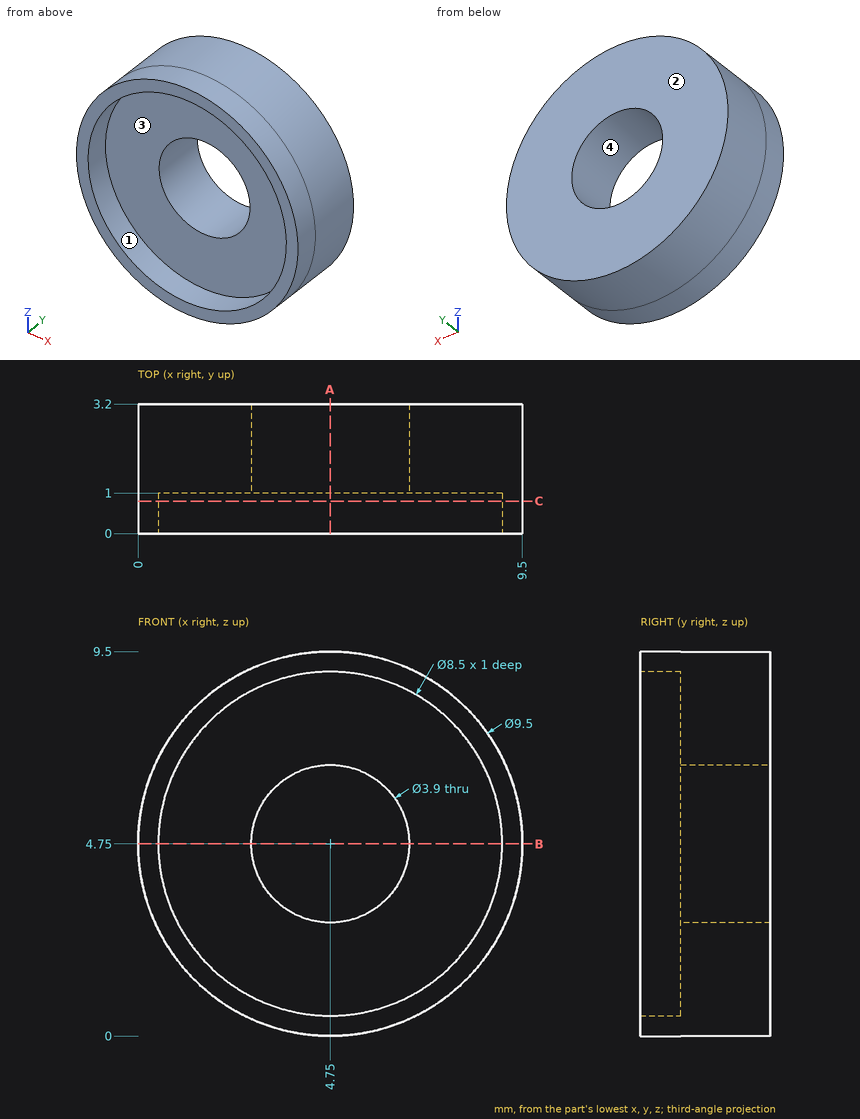
Check sheet for the drawn part. Datum: minimum x, y, z corner. Units: mm. A direction names the side the tool comes from. Round coordinates to 2 decimals unless told otherwise and drop trailing zeros. Loops run counter-clockwise (first coordinate to the right, second up) from the corner with the lowest first, then second, coordinate; pieces in that order, holes last. Notation, with made-up numbers: M 35.25,17.25 L 84.25,17.25 A27 ccw 84.25,36.25 Z; hole C 11,8.25 d7. An arc over 180 degrees is marked long. One line per question, with ' | ' between items. Start each with the question number.
Item 1: Scan lines: probe 1 along X at (y, z) = (0.4, 4.75); probe 2 along X at (y, z) = (1.5, 4.75); probe 3 along Y at (x, z) = (2.5, 7.75). Record each from-to range of solid material in increasing order.
Item 2: Release check for a two-part mould opening along X. For the marked faces 1 and 2 record: released by +X, released by -X, zero draft, split by the parting line, or undercut.
Item 3: Gauge pin test, flat ends, axial feed: pin 1 Ø1 at (x, y) = (7.5, 0.5) entering from +Z; pin 2 Ø3.5 at (x, z) = (4.75, 4.75) entering from -Y. Record the tip position at first contact, or that the pin passes through.
Item 4: Section check A-A (x = 4.75). Record the boundary of the cut face in (y, z), and give its area (3 significant figures).
Item 5: Section check C-C (y = 0.8). Record the boundary of the cut face in (x, z).
Item 6: Section check B-B (z = 4.75). Record the boundary of the cut face in (x, y).
Item 7: Set-up check for the marked faces 3 and 4: record each of +Z, -Z, +X, -X, +Y, -Y from which the full face is reachable in a straight line by a thin tool's end or side.
Worked out:
1) probe 1: 0 to 0.5, 9 to 9.5 | probe 2: 0 to 2.8, 6.7 to 9.5 | probe 3: 1 to 3.2
2) face 1: undercut | face 2: zero draft
3) pin 1: z = 8.93 | pin 2: through
4) outline: M 0,0 L 3.2,0 L 3.2,2.8 L 1,2.8 L 1,0.5 L 0,0.5 Z; M 0,9 L 1,9 L 1,6.7 L 3.2,6.7 L 3.2,9.5 L 0,9.5 Z | area: 13.3 mm^2
5) outline: C 4.75,4.75 d9.5; hole C 4.75,4.75 d8.5
6) outline: M 0,0 L 0.5,0 L 0.5,1 L 2.8,1 L 2.8,3.2 L 0,3.2 Z; M 6.7,1 L 9,1 L 9,0 L 9.5,0 L 9.5,3.2 L 6.7,3.2 Z
7) face 3: -Y | face 4: +Y, -Y
